from build123d import *

# Parameters (mm, degrees)
F0_R     = 6
F1_DEPTH = 12.5
F2_W     = 28
F2_H     = 19
F3_DEPTH = 8


with BuildPart() as f1:
    # F0 (on Top) → F1 (new body)
    with BuildSketch(Plane.XY):
        Circle(F0_R)
    extrude(amount=F1_DEPTH)

    # F2 (on Right) → F3 (join, symmetric)
    with BuildSketch(Plane.YZ):
        with Locations((0, -9.5)):
            Rectangle(F2_W, F2_H)
    extrude(amount=F3_DEPTH, both=True)

    # F2 (on Right) → F4 (revolve)
    with BuildSketch(Plane.YZ):
        with BuildLine():
            ThreePointArc((0, 15.9491937459), (1.8805486292, 15.4010638062), (3.1720772546, 13.9283576619))
            Line((3.1720772546, 13.9283576619), (4.0744187722, 14.3593794546))
            Line((4.0744187722, 14.3593794546), (4.0744187722, 34.3593794546))
            Line((4.0744187722, 34.3593794546), (3.5, 34.3593794546))
            add(Edge.make_bspline(
                [(0, 32.6093794546), (3.5, 32.6093794546), (3.5, 34.3593794546)],
                knots=[4.7123889804, 4.7123889804, 4.7123889804, 6.2831853072, 6.2831853072, 6.2831853072], degree=2, weights=[1, 0.7071067812, 1]))
            Line((0, 32.6093794546), (0, 15.9491937459))
        make_face()
        with BuildLine():
            Line((0, 12.4491937459), (3.5, 12.4491937459))
            ThreePointArc((3.5, 12.4491937459), (3.4170360249, 13.2067323946), (3.1720772546, 13.9283576619))
            ThreePointArc((3.1720772546, 13.9283576619), (1.8805486292, 15.4010638062), (0, 15.9491937459))
            Line((0, 15.9491937459), (0, 12.4491937459))
        make_face()
        with BuildLine():
            Line((0, 34.3593794546), (0, 32.6093794546))
            add(Edge.make_bspline(
                [(0, 32.6093794546), (3.5, 32.6093794546), (3.5, 34.3593794546)],
                knots=[4.7123889804, 4.7123889804, 4.7123889804, 6.2831853072, 6.2831853072, 6.2831853072], degree=2, weights=[1, 0.7071067812, 1]))
            Line((3.5, 34.3593794546), (0, 34.3593794546))
        make_face()
        with BuildLine():
            Line((0, 36.1093794546), (0, 34.3593794546))
            Line((0, 34.3593794546), (3.5, 34.3593794546))
            add(Edge.make_bspline(
                [(3.5, 34.3593794546), (3.5, 36.1093794546), (0, 36.1093794546)],
                knots=[0, 0, 0, 1.5707963268, 1.5707963268, 1.5707963268], degree=2, weights=[1, 0.7071067812, 1]))
        make_face()
        with BuildLine():
            ThreePointArc((0, 8.9491937459), (2.4748737342, 9.9743200117), (3.5, 12.4491937459))
            Line((3.5, 12.4491937459), (0, 12.4491937459))
            Line((0, 12.4491937459), (0, 8.9491937459))
        make_face()
    revolve(axis=Axis((0, 0, 25.1542866002), (0, 0, -1)))


solid = f1.part
Source: CAD feature listing. Evaluate the final solid. Frame: model axes, mm. A direction names the side the tool comes from. Round coordinates to 2 decimals unless told otherwise and drop trailing zeros. Order: outer loops, then holes, each group sorted by start corner. A loop starts at its lowest first (then second) coordinate and runs counter-clockwise, first axis right, second up. Notation, with made-up numbers: (-31, 12.25) - (-24, 12.25) arc R21 cw to (-24, 38.25) - close; hole circle Ø4 at (67.5, 10.5). An arc over 180 degrees is marked (long way). Use a Markdown table: item, result. Add a question column.
1. First-contact query: pin 1 (8 mm diameter, centred on x = 5, y = 2, fed in from +Z); pin 2 (5 mm diameter, centred on x = 0, y = -4, fed in from +Z); pin 3 (6 mm diameter, centred on y = 4.5, z = 11.5, fed in from -X). Flat tips, straight axial feed; report the tip coordinate or a pass-through.
2. Set-up query: faces 1 (the cylindrical face through (2.754, -3.003, 24.499)), 2 (the flat face through (0, 0, -19)). Return all of +Z, -Z, +X, -X, +Y, -Y with unobstructed straight access to the full face (end or side cutting, diameter ignored); none if empty.
3. Section query C-C (y = 11). Return the cut outline in (x, z), then the cut area to 3 significant figures.
4. Section query D-D (z = 32). Return the cut outline in (x, y), then the cut area to 3 significant figures.
5. Section query B-B (z = 4). Return the cut outline in (x, y), then the cut area to 3 significant figures.
6. Line query: probe 1 along Z at (x, y) = (5.5, 0.5); probe 2 along Z at (x, y) = (-6.5, -3.25); probe 3 along Z at (x, y) = (-2.75, 2.25). Output: solid intervals per line, ascending.
7. Section query A-A (y = 5). Return the cut outline in (x, z), then the cut area to 3 significant figures.
8. Mould query, pull axis Z, two halves, no side actions, for faces 3 (the flat face through (5.4, -3.3, 0)), 4 (the flat face through (0, -14, -10)), 5 (the flat face through (3, -3, 12.5)). Classes: +Z half, -Z half, draft (parallel to the pull), parting line (faces both ways), or undercut.
Derived:
| question | item | result |
|---|---|---|
| 1 | pin 1 | z = 35.97 |
| 1 | pin 2 | z = 35.94 |
| 1 | pin 3 | x = -5.81 |
| 2 | face 1 | +Z |
| 2 | face 2 | -Z, +X, -X, +Y, -Y |
| 3 | outline | (-8, -19) - (8, -19) - (8, 0) - (-8, 0) - close |
| 3 | area | 304 mm2 |
| 4 | outline | circle Ø8.15 at (0, 0) |
| 4 | area | 52.2 mm2 |
| 5 | outline | circle Ø12 at (0, 0) |
| 5 | area | 113 mm2 |
| 6 | probe 1 | -19 to 12.5 |
| 6 | probe 2 | -19 to 0 |
| 6 | probe 3 | -19 to 12.5, 14.11 to 34.36 |
| 7 | outline | (-8, -19) - (8, -19) - (8, 0) - (3.32, 0) - (3.32, 12.5) - (-3.32, 12.5) - (-3.32, 0) - (-8, 0) - close |
| 7 | area | 387 mm2 |
| 8 | face 3 | +Z half |
| 8 | face 4 | draft |
| 8 | face 5 | undercut |
